```python
from build123d import *

# Parameters (mm, degrees)
SKETCH1_W           = 110
SKETCH1_H           = 30
BOSS_EXTRUDE1_DEPTH = 12
FILLET2_R           = 8
SKETCH4_R           = 6.5
CUT_EXTRUDE1_DEPTH  = 67.870108383
SKETCH3_W           = 23
SKETCH3_H           = 13
CUT_EXTRUDE2_DEPTH  = 10
SKETCH5_W           = 32
SKETCH5_H           = 18
CUT_EXTRUDE3_DEPTH  = 1.5
FILLET4_R           = 3
SKETCH6_R           = 1
CUT_EXTRUDE4_DEPTH  = 4


with BuildPart() as part:
    # Sketch1 → Boss-Extrude1 (new body)
    with BuildSketch(Plane(origin=(0, 0, 0), x_dir=(1, 0, 0), z_dir=(0, 1, 0))):
        with Locations((8.243243243, 3.108108108)):
            Rectangle(SKETCH1_W, SKETCH1_H)
    extrude(amount=BOSS_EXTRUDE1_DEPTH)

    # Fillet2
    fillet2_edges = [part.edges().sort_by_distance(p)[0] for p in [
        (-46.756756757, 6, -18.108108108),
        (63.243243243, 6, -18.108108108),
        (63.243243243, 6, 11.891891892),
        (-46.756756757, 6, 11.891891892),
    ]]
    fillet(fillet2_edges, radius=FILLET2_R)

    # Sketch4 → Cut-Extrude1 (cut, through all)
    with BuildSketch(Plane(origin=(0, 12, 0), x_dir=(1, 0, 0), z_dir=(0, 1, 0))):
        with Locations(Location((-27.929103529, 3.108108108, 0), (0, 0, 270))):
            Circle(SKETCH4_R)
    extrude(amount=-CUT_EXTRUDE1_DEPTH, mode=Mode.SUBTRACT)

    # Sketch3 → Cut-Extrude2 (cut)
    with BuildSketch(Plane(origin=(0, 12, 0), x_dir=(1, 0, 0), z_dir=(0, 1, 0))):
        with Locations((-23.179103529, 3.108108108)):
            Rectangle(SKETCH3_W, SKETCH3_H)
    extrude(amount=-CUT_EXTRUDE2_DEPTH, mode=Mode.SUBTRACT)

    # Sketch5 → Cut-Extrude3 (cut)
    with BuildSketch(Plane(origin=(0, 12, 0), x_dir=(1, 0, 0), z_dir=(0, 1, 0))):
        with Locations((-23.262280593, 3.273133416)):
            Rectangle(SKETCH5_W, SKETCH5_H)
    extrude(amount=-CUT_EXTRUDE3_DEPTH, mode=Mode.SUBTRACT)

    # Fillet4
    fillet4_edges = [part.edges().sort_by_distance(p)[0] for p in [
        (-39.262280593, 11.25, 5.726866584),
        (-39.262280593, 11.25, -12.273133416),
        (-7.262280593, 11.25, -12.273133416),
        (-7.262280593, 11.25, 5.726866584),
    ]]
    fillet(fillet4_edges, radius=FILLET4_R)

    # Sketch6 → Cut-Extrude4 (cut)
    with BuildSketch(Plane(origin=(0, 10.5, 0), x_dir=(1, 0, 0), z_dir=(0, 1, 0))):
        with Locations(Location((-37.179103529, 3.108108108, 0), (0, 0, 270))):
            Circle(SKETCH6_R)
        with Locations(Location((-9.179103529, 3.108108108, 0), (0, 0, 90))):
            Circle(SKETCH6_R)
    extrude(amount=-CUT_EXTRUDE4_DEPTH, mode=Mode.SUBTRACT)


solid = part.part
```
Geometry: final body of the model. Coordinates: model frame, mm. A direction names the side the tool comes from. Coordinates: 2 decimals unless noted, no trailing zeros. Order: outer loops, then holes, each group sorted by start corner. A loop starts at its lowest first (then second) coordinate and runs counter-clockwise, first axis right, second up. Notation, with made-up numbers: (40, -39.5) -> (94, -39.5) arc R35 cw to (94, -6.5) -> close; hole circle Ø10 at (74.25, -1). An arc over 180 degrees is marked (long way). Answer in a Markdown table with one row per item.
Item 1: Ray query, L1, parallel to X at y = 10, z = -9.5; L2, parallel to Z at x = -30.5, y = 11; L3, parallel to Y at x = -27.5, z = -10. Return the intervals inside material, ascending.
Return value:
| item | result |
|---|---|
| L1 | x = -46.76 to -34.68, -11.68 to 63.24 |
| L2 | z = -18.11 to -12.27, 5.73 to 11.89 |
| L3 | y = 0 to 10.5 |
Item 2: Section C-C on z = -6. Output: boundary loops of the cut face in (x, y).
Return value:
| item | result |
|---|---|
| outline | (-46.76, 0) -> (-33.75, 0) -> (-33.75, 2) -> (-34.68, 2) -> (-34.68, 10.5) -> (-39.26, 10.5) -> (-39.26, 12) -> (-46.76, 12) -> close; (-22.11, 0) -> (63.24, 0) -> (63.24, 12) -> (-7.26, 12) -> (-7.26, 10.5) -> (-11.68, 10.5) -> (-11.68, 2) -> (-22.11, 2) -> close |
Item 3: Section D-D on y = 9.25. Output: boundary loops of the cut face in (x, z), plus the area to 3 significant figures.
Return value:
| item | result |
|---|---|
| outline | (-46.76, -10.11) arc R8 ccw to (-38.76, -18.11) -> (55.24, -18.11) arc R8 ccw to (63.24, -10.11) -> (63.24, 3.89) arc R8 ccw to (55.24, 11.89) -> (-38.76, 11.89) arc R8 ccw to (-46.76, 3.89) -> close; hole circle Ø2 at (-37.18, -3.11); hole (-34.68, -9.61) -> (-11.68, -9.61) -> (-11.68, 3.39) -> (-34.68, 3.39) -> close; hole circle Ø2 at (-9.18, -3.11) |
| area | 2,940 mm² |
Item 4: Contact query for flat-ended pins moving along their axis: P1, Ø5, axis at y = 1.5, z = 8, coming from the -X side; P2, Ø2, axis at x = -37.5, z = -3, coming from the +Y side; P3, Ø1.2, axis at x = -9.18, z = -3.11, coming from the +Y side. Output: stop coordinate, or through.
Return value:
| item | result |
|---|---|
| P1 | stops at x = -46.59 |
| P2 | stops at y = 10.5 |
| P3 | stops at y = 6.5 |
Item 5: Section A-A on y = 3.25. Output: boundary loops of the cut face in (x, z).
Return value:
| item | result |
|---|---|
| outline | (-46.76, -10.11) arc R8 ccw to (-38.76, -18.11) -> (55.24, -18.11) arc R8 ccw to (63.24, -10.11) -> (63.24, 3.89) arc R8 ccw to (55.24, 11.89) -> (-38.76, 11.89) arc R8 ccw to (-46.76, 3.89) -> close; hole (-34.68, -9.61) -> (-11.68, -9.61) -> (-11.68, 3.39) -> (-34.68, 3.39) -> close |
Item 6: Section B-B on x = -29. Output: boundary loops of the cut face in (y, z).
Return value:
| item | result |
|---|---|
| outline | (0, -18.11) -> (12, -18.11) -> (12, -12.27) -> (10.5, -12.27) -> (10.5, -9.61) -> (2, -9.61) -> (2, -9.52) -> (0, -9.52) -> close; (0, 3.3) -> (2, 3.3) -> (2, 3.39) -> (10.5, 3.39) -> (10.5, 5.73) -> (12, 5.73) -> (12, 11.89) -> (0, 11.89) -> close |
Item 7: Access query for faces 1 (the flat face through (8, 6, 11.892)), 2 (the flat face through (-23, 6, -9.608)). Directions: +Z, -Z, +X, -X, +Y, -Y. A direction counts if a zero-diameter tool reaches every point of the face in a straight line with its end or side. Return the directions, or none.
Return value:
| item | result |
|---|---|
| face 1 | +Z, +X, -X, +Y, -Y |
| face 2 | +Y |
Item 8: Draft query along X for faces 3 (the cylindrical face through (-26, 1, 3.1)), 4 (the flat face through (8, 6, -18.108)), 5 (the cylindrical face through (60.962, 6.084, -15.702)). Return one class per face: released by +X, released by -X, zero draft, split by the parting line, or undercut.
Return value:
| item | result |
|---|---|
| face 3 | undercut |
| face 4 | zero draft |
| face 5 | released by +X |
